Verification items for the finished model (mm, model axes). A direction names the side the tool comes from. Give positions to 0.01 mm unless a question says otherwise; leave off trailing zeros. Loops run counter-clockwise (first coordinate to the right, second up) from the corner with the lowest first, then second, coordinate; pieces in that order, holes last. Notation, with made-up numbers: M -17.5,-24 L 28.5,-24 A33 ccw 28.5,13 Z; hole C 14.5,-32 d4. An arc over 180 degrees is marked long. Use CSV: the item, a comma, the result in double quotes.
Autodesk Inventor part; units mm, degrees
ref_plane "YZ Plane" through (0, 0, 0) normal (1, 0, 0) x (0, 1, 0)
ref_plane "XZ Plane" through (0, 0, 0) normal (0, 1, 0) x (-1, 0, 0)
ref_plane "XY Plane" through (0, 0, 0) normal (0, 0, 1) x (1, 0, 0)
sketch "Sketch1" plane through (0, 0, 0) normal (0, 0, 1) x (1, 0, 0)
  line L0 (0, 0) -> (335, 0)
  line L1 (335, 0) -> (335, 300)
  line L2 (335, 300) -> (0, 300)
  line L3 (0, 300) -> (0, 0)
  dimension "d0" = 335
  dimension "d1" = 300
extrude "Plate" add sketch "Sketch1" along normal blind 10.5
sketch "Sketch3" plane through (0, 0, 10.5) normal (0, 0, 1) x (1, 0, 0)
  circle A0 centre (316.15, 18.85) radius 7.85
  line L0 (335, 0) -> (335, 300)
  line L1 (0, 0) -> (335, 0)
  circle A1 centre (316.15, 18.85) radius 4
  line L2 (0, 300) -> (0, 0)
  line L3 (335, 300) -> (0, 300)
  circle A2 centre (18.85, 199.55) radius 7.85
  circle A3 centre (100.45, 281.15) radius 7.85
  point P0 (18.85, 18.85)
  point P1 (316.15, 281.15)
  dimension "d4" = 15.7
  dimension "d5" = 18.85
  dimension "d6" = 18.85
  dimension "d7" = 8
  dimension "d8" = 18.85
  dimension "d9" = 18.85
  dimension "d10" = 18.85
  dimension "d11" = 18.85
  dimension "d19" = 18.85
  dimension "d20" = 18.85
  dimension "d21" = 15.7
  dimension "d22" = 15.7
  dimension "d23" = 180.7
  dimension "d24" = 215.7
hole "Small screw" at (18.85, 18.85, 10.5) at (316.15, 281.15, 10.5) at (316.15, 18.85, 10.5) at (18.85, 199.55, 10.5) at (100.45, 281.15, 10.5) direction (0, 0, -1) diameter 8 end through all countersink diameter 15.7 countersink angle 90
sketch "Sketch4" plane through (0, 0, 10.5) normal (0, 0, 1) x (1, 0, 0)
  circle A0 centre (100.45, 281.15) radius 7.85
  circle A1 centre (18.85, 199.55) radius 7.85
  circle A2 centre (18.85, 239.15) radius 11.75
  circle A3 centre (60.85, 281.15) radius 11.75
  circle A4 centre (18.85, 199.55) radius 4
  circle A5 centre (18.85, 199.55) radius 7.85
  point P0 (0, 0)
  dimension "d25" = 23.5
  dimension "d26" = 23.5
  dimension "d27" = 0
  dimension "d28" = 0
  dimension "d29" = 39.6
  dimension "d30" = 15.7
  dimension "d31" = 39.6
hole "Big screw" at (60.85, 281.15, 10.5) at (18.85, 239.15, 10.5) direction (0, 0, -1) diameter 12 end through all countersink diameter 23.5 countersink angle 90
fillet "Stor runding" radius 40 1 edges at (0, 300, 5.25)
sketch "Sketch6" plane through (0, 0, 10.5) normal (0, 0, 1) x (1, 0, 0)
  arc A0 (40, 300) -> (0, 260) centre (40, 260) ccw
  line L0 (0, 260) -> (0, 0)
  line L1 (0, 0) -> (335, 0)
  line L2 (335, 0) -> (335, 300)
  line L3 (335, 300) -> (40, 300)
  circle A1 centre (18.85, 239.15) radius 11.75
  circle A2 centre (60.85, 281.15) radius 11.75
  circle A3 centre (100.45, 281.15) radius 7.85
  circle A4 centre (18.85, 199.55) radius 7.85
  circle A5 centre (316.15, 18.85) radius 7.85
  circle A6 centre (316.15, 281.15) radius 7.85
  circle A7 centre (18.85, 18.85) radius 7.85
  line L4 (17.5207, 293.0859) -> (6.9141, 282.4793)
  line L5 (6.9141, 282.4793) -> (57.8257, 231.5676)
  line L6 (57.8257, 231.5676) -> (68.4324, 242.1743)
  line L7 (68.4324, 242.1743) -> (17.5207, 293.0859)
  arc A8 (40, 300) -> (0, 260) centre (40, 260) ccw
  dimension "d40" = 15
  dimension "d41" = 72
  dimension "d42" = 135
extrude "Extrusion2" cut sketch "Sketch6" against normal up to next contours L4 A0 | L7 L6 L5 L4
fillet "Fillet2" radius 7.5 2 edges at (68.4324, 242.1743, 5.25) (57.8257, 231.5676, 5.25)
sketch "Sketch7" plane through (0, 0, 0) normal (0, 0, -1) x (-1, 0, 0)
  circle A0 centre (-116, 184) radius 74.5
  circle A1 centre (-116, 250) radius 4.5
  circle A2 centre (-182, 184) radius 4.5
  circle A3 centre (-116, 118) radius 4.5
  circle A4 centre (-116, 118) radius 4.5
  circle A5 centre (-50, 184) radius 4.5
  point P0 (0, 0)
extrude "Extrusion3" cut sketch "Sketch7" against normal up to next contours A1 | A2 | A3 | A5
equation "\"d5\" = d6"
equation "\"d21\" = d4"
equation "\"d22\" = d21"
equation "\"d31\" = d29"
properties part number "Mount plate UR"
(1) Section check D-D on x = 182. Record the cut outline in (y, z), plus the area to 3 significant figures.
Calculated:
outline,"M 0,0 L 179.5,0 L 179.5,10.5 L 0,10.5 Z; M 188.5,0 L 300,0 L 300,10.5 L 188.5,10.5 Z"
area,"3,060 mm²"
(2) Depth check by flat-ended pin: pin 1 Ø8 at (x, y) = (116, 118) entering from -Z; pin 2 Ø15.5 at (x, y) = (60.85, 281.15) entering from +Z. Enter the tip coordinate at first touch or a pass-through.
Calculated:
pin 1,"passes through"
pin 2,"stops at z = 6.5"
(3) Section check A-A on x = 116. Record the cut outline in (y, z).
Calculated:
outline,"M 0,0 L 113.5,0 L 113.5,10.5 L 0,10.5 Z; M 122.5,0 L 245.5,0 L 245.5,10.5 L 122.5,10.5 Z; M 254.5,0 L 300,0 L 300,10.5 L 254.5,10.5 Z"
(4) Section check B-B on y = 184. Record the cut outline in (x, z), plus the area to 3 significant figures.
Calculated:
outline,"M 0,0 L 45.5,0 L 45.5,10.5 L 0,10.5 Z; M 54.5,0 L 177.5,0 L 177.5,10.5 L 54.5,10.5 Z; M 186.5,0 L 335,0 L 335,10.5 L 186.5,10.5 Z"
area,"3,330 mm²"
(5) Section check C-C on y = 118. Record the cut outline in (x, z).
Calculated:
outline,"M 0,0 L 111.5,0 L 111.5,10.5 L 0,10.5 Z; M 120.5,0 L 335,0 L 335,10.5 L 120.5,10.5 Z"
(6) Tool access check on faces 5 (the conical face through (100.6, 285.4, 6.9)), 6 (the flat face through (29.399, 259.994, 5.324)). Record the directions out of +Z, -Z, +X, -X, +Y, -Y that give a thin tool (end or side, any length) a straight path to the whole face; none if there is none.
Calculated:
face 5,"+Z"
face 6,"+Z, -Z"
(7) Scan lines: L1, parallel to Y at x = 116, z = 7; L2, parallel to Y at x = 182, z = 7; L3, parallel to Y at x = 27, z = 10 (3 decimals). Record each from-to range of solid material in increasing order. Write a range as from..to.
Calculated:
L1,"y = 0..113.5, 122.5..245.5, 254.5..300"
L2,"y = 0..179.5, 188.5..300"
L3,"y = 0..231.395, 246.905..262.393, 283.607..297.829"
(8) Mould release check, pull along X, two halves, no side actions. Record for faces 1 (the conical face through (21.7, 22, 6.9)), 2 (the cylindrical face through (312.184, 19.371, 3.278)), 3 (the flat face through (165, 0, 5)), 4 (the flat face through (335, 148, 5)): released by +X, released by -X, zero draft, split by the parting line, or undercut.
Calculated:
face 1,"undercut"
face 2,"undercut"
face 3,"zero draft"
face 4,"released by +X"
